```python
from build123d import *

# Parameters (mm, degrees)
SKETCH_1_R          = 8.75
SKETCH_1_R_2        = 1.8
EXTRUDE_1_DEPTH     = 6.4
SKETCH_7_R          = 3
CUT_EXTRUDE_1_DEPTH = 3.2
SKETCH_8_R          = 4
SKETCH_8_R_2        = 1.8
EXTRUDE_2_DEPTH     = 5
SKETCH_9_R          = 5.65
SKETCH_9_R_2        = 4
CUT_EXTRUDE_2_DEPTH = 2


with BuildPart() as part:
    # Эскиз1 → Бобышка-Вытянуть1 (new body)
    with BuildSketch(Plane(origin=(0, 0, 0), x_dir=(1, 0, 0), z_dir=(0, 1, 0))):
        with Locations((-1.25, 0)):
            Circle(SKETCH_1_R)
        Circle(SKETCH_1_R_2, mode=Mode.SUBTRACT)
    extrude(amount=EXTRUDE_1_DEPTH)

    # Эскиз7 → Вырез-Вытянуть1 (cut)
    with BuildSketch(Plane(origin=(0, 6.4, 0), x_dir=(1, 0, 0), z_dir=(0, 1, 0))):
        Circle(SKETCH_7_R)
    extrude(amount=-CUT_EXTRUDE_1_DEPTH, mode=Mode.SUBTRACT)

    # Эскиз8 → Бобышка-Вытянуть2 (add)
    with BuildSketch(Plane.XZ):
        Circle(SKETCH_8_R)
        Circle(SKETCH_8_R_2, mode=Mode.SUBTRACT)
    extrude(amount=EXTRUDE_2_DEPTH)

    # Эскиз9 → Вырез-Вытянуть2 (cut)
    with BuildSketch(Plane.XZ):
        Circle(SKETCH_9_R)
        Circle(SKETCH_9_R_2, mode=Mode.SUBTRACT)
    extrude(amount=-CUT_EXTRUDE_2_DEPTH, mode=Mode.SUBTRACT)


solid = part.part
```
Verification items for the finished model (mm, model axes). A direction names the side the tool comes from. Round coordinates to 2 decimals unless told otherwise and drop trailing zeros. Write each loop counter-clockwise with the first axis right and the second up, starting at its lowest first coordinate (ties: lowest second). Pieces come first, ordered by that corner, then holes.
1. Gauge pin test, flat ends, axial feed: P1, Ø4, axis at x = 2, y = -4, coming from the -Z side; P2, Ø3, axis at x = -0.5, z = 1, coming from the +Y side; P3, Ø3, axis at x = 0, z = 0, coming from the +Y side; P4, Ø1.5, axis at x = -4, y = 4, coming from the +Z side. Record the tip position at first contact, or that the pin passes through.
2. Access from +Z, -Z, +X, -X, +Y, -Y to the whole of each face (thin tool, end or side, straight path). Record for faces 5 (the cylindrical face through (-3, 5, 0)), 6 (the flat face through (-3.3, 6.4, -0.1)), 7 (the flat face through (2, 2, -4)).
3. Section check A-A on z = 0. Enter the section's corners in (x, y), plus the area to 3 significant figures.
4. Section check C-C on x = -1.25. Enter the section's corners in (y, z).
5. Section check B-B on y = 1. Enter the section's corners in (x, z).
6. Draft check along Z on faces 1 (the cylindrical face through (-8.194, 3.155, 5.324)), 2 (the flat face through (-5, 0, 4)), 3 (the flat face through (0, 3.2, 2)), 4 (the cylindrical face through (5.39, 0.99, 1.7)). Enter one of: +Z half, -Z half, draft (parallel to the pull), parting line (faces both ways), or undercut.
7. Section check D-D on z = -4.75. Enter the section's corners in (x, y).
8. Scan lines: L1, parallel to X at y = 4.75, z = 0; L2, parallel to Z at x = 0, y = -1.75; L3, parallel to Z at x = 0, y = 0.5. Record each from-to range of solid material in increasing order.
Answer:
1. P1: stops at z = -4
1. P2: stops at y = 3.2
1. P3: passes through
1. P4: stops at z = 8.52
2. face 5: +Y
2. face 6: +Z, -Z, +X, -X, +Y
2. face 7: -Y
3. outline: (-10, 0) - (-5.65, 0) - (-5.65, 2) - (-4, 2) - (-4, -5) - (-1.8, -5) - (-1.8, 3.2) - (-3, 3.2) - (-3, 6.4) - (-10, 6.4) - close; (1.8, -5) - (4, -5) - (4, 2) - (5.65, 2) - (5.65, 0) - (7.5, 0) - (7.5, 6.4) - (3, 6.4) - (3, 3.2) - (1.8, 3.2) - close
3. area: 96.7 mm2
4. outline: (-5, -3.8) - (2, -3.8) - (2, -5.51) - (0, -5.51) - (0, -8.75) - (6.4, -8.75) - (6.4, -2.73) - (3.2, -2.73) - (3.2, -1.3) - (-5, -1.3) - close; (-5, 1.3) - (3.2, 1.3) - (3.2, 2.73) - (6.4, 2.73) - (6.4, 8.75) - (0, 8.75) - (0, 5.51) - (2, 5.51) - (2, 3.8) - (-5, 3.8) - close
5. outline: circle Ø17.5 at (-1.25, 0); circle Ø8 at (0, 0); hole circle Ø11.3 at (0, 0); hole circle Ø3.6 at (0, 0)
6. face 1: parting line
6. face 2: draft
6. face 3: undercut
6. face 4: undercut
7. outline: (-8.6, 0) - (-3.06, 0) - (-3.06, 2) - (3.06, 2) - (3.06, 0) - (6.1, 0) - (6.1, 6.4) - (-8.6, 6.4) - close
8. L1: x = -10 to -3, 3 to 7.5
8. L2: z = -4 to -1.8, 1.8 to 4
8. L3: z = -8.66 to -5.65, -4 to -1.8, 1.8 to 4, 5.65 to 8.66
